from build123d import *

# Parameters (mm, degrees)
SKETCH1_R           = 17
BOSS_EXTRUDE1_DEPTH = 1
SKETCH2_W           = 18.565645136
SKETCH2_H           = 14.338667356
BOSS_EXTRUDE2_DEPTH = 4
SKETCH3_R           = 11.539294854
BOSS_EXTRUDE3_DEPTH = 1


with BuildPart() as part:
    # Sketch1 → Boss-Extrude1 (new body)
    with BuildSketch(Plane(origin=(0, 0, 0), x_dir=(1, 0, 0), z_dir=(0, 1, 0))):
        with Locations(Location((0, 0, 0), (0, 0, 270))):
            Circle(SKETCH1_R)
    extrude(amount=BOSS_EXTRUDE1_DEPTH)

    # Sketch2 → Boss-Extrude2 (add)
    with BuildSketch(Plane.XZ):
        with Locations((3.402156218, -2.462998516)):
            Rectangle(SKETCH2_W, SKETCH2_H)
    extrude(amount=BOSS_EXTRUDE2_DEPTH)

    # Sketch3 → Boss-Extrude3 (add)
    with BuildSketch(Plane(origin=(0, 1, 0), x_dir=(1, 0, 0), z_dir=(0, 1, 0))):
        with Locations(Location((0, 0, 0), (0, 0, 270))):
            Circle(SKETCH3_R)
    extrude(amount=BOSS_EXTRUDE3_DEPTH)


solid = part.part
The listing builds one solid part. Answer for the finished solid, in the listing's coordinates (mm). A direction names the side the tool comes from. Round coordinates to 2 decimals unless told otherwise and drop trailing zeros. Order: outer loops, then holes, each group sorted by start corner. A loop starts at its lowest first (then second) coordinate and runs counter-clockwise, first axis right, second up. Notation, with made-up numbers: (17, 84.5) -> (21, 84.5) arc R23 ccw to (21, 115.5) -> close; hole circle Ø6 at (13, 58.25). An arc over 180 degrees is marked (long way). Put each result on its own line as item: value.
Q1. Section C-C, the plane y = 0.6 is taken. Write down the section's boundary in (x, z), and give its area (3 significant figures).
Results list:
outline: circle Ø34 at (0, 0)
area: 908 mm^2
Q2. Section D-D, the plane y = -1.8 is taken. Write down the section's boundary in (x, z).
Results list:
outline: (-5.88, -9.63) -> (12.68, -9.63) -> (12.68, 4.71) -> (-5.88, 4.71) -> close
Q3. Consider line 1 along Z through (x, y) = (6.5, -2.15); line 2 along X through (y, z) = (-3.5, -7.5); line 3 along Y through (x, z) = (-1, 10). Determine where each line is inside the solid, lowest interval first.
Results list:
line 1: -9.63 to 4.71
line 2: -5.88 to 12.68
line 3: 0 to 2
Q4. Section B-B, the plane z = 0 is taken. Write down the section's boundary in (x, y), and give its area (3 significant figures).
Results list:
outline: (-17, 0) -> (-5.88, 0) -> (-5.88, -4) -> (12.68, -4) -> (12.68, 0) -> (17, 0) -> (17, 1) -> (11.54, 1) -> (11.54, 2) -> (-11.54, 2) -> (-11.54, 1) -> (-17, 1) -> close
area: 131 mm^2
Q5. Each of these flat-tipped pins is pushed along its axis until it touches: P1, Ø3, axis at x = 2.5, y = -1, coming from the +Z side; P2, Ø1.5, axis at y = 0.5, z = 9.5, coming from the +X side; P3, Ø1.5, axis at x = -10, y = -2, coming from the +Z side; P4, Ø1.2, axis at y = -1.5, z = -3, coming from the +X side (3 decimals). Where does it stop, or does it pass through?
Results list:
P1: z = 16.94
P2: x = 14.58
P3: through
P4: x = 12.685
Q6. Section A-A, the plane x = 0 is taken. Write down the section's boundary in (y, z), and give its area (3 significant figures).
Results list:
outline: (-4, -9.63) -> (0, -9.63) -> (0, -17) -> (1, -17) -> (1, -11.54) -> (2, -11.54) -> (2, 11.54) -> (1, 11.54) -> (1, 17) -> (0, 17) -> (0, 4.71) -> (-4, 4.71) -> close
area: 114 mm^2
Q7. Which of the six approach directions +Z, -Z, +X, -X, +Y, -Y give full straight-line access (tool end or side, diameter ignored) to faces 1 (the flat face through (12.685, -2, -3)), 2 (the flat face through (3, -2, 4.706)), 3 (the flat face through (-11, 1, 4)), 4 (the flat face through (3, -2, -9.632))?
Results list:
face 1: +Z, -Z, +X, -Y
face 2: +Z, +X, -X, -Y
face 3: +Y
face 4: -Z, +X, -X, -Y
